```python
from build123d import *

# Parameters (mm, degrees)
SKETCH3_R           = 3
CUT_EXTRUDE1_DEPTH  = 1.5
SKETCH4_R           = 1.5
CUT_EXTRUDE2_DEPTH  = 2.5
SKETCH5_R           = 5
SKETCH5_R_2         = 4
EXTRUDE_THIN1_DEPTH = 2


with BuildPart() as part:
    # Sketch1 → Revolve1 (revolve)
    with BuildSketch(Plane(origin=(0, 0, 0), x_dir=(1, 0, 0), z_dir=(0, 1, 0))):
        Polygon((0, -1), (4.5, -1), (4.5, 0), (7.5, 0), (7.5, -1), (14, -1), (14, 1), (15, 1), (15, 2), (0, 2), align=None)
    revolve(axis=Axis((0, 0, -2), (0, 0, 1)))

    # Sketch3 → Cut-Extrude1 (cut)
    with BuildSketch(Plane.XY.offset(1)):
        Circle(SKETCH3_R)
    extrude(amount=-CUT_EXTRUDE1_DEPTH, mode=Mode.SUBTRACT)

    # Sketch4 → Cut-Extrude2 (cut, through all)
    with BuildSketch(Plane.XY.offset(-0.5)):
        Circle(SKETCH4_R)
    extrude(amount=-CUT_EXTRUDE2_DEPTH, mode=Mode.SUBTRACT)

    # Sketch5 → Extrude-Thin1 (add)
    with BuildSketch(Plane(origin=(0, 0, -2), x_dir=(-1, 0, 0), z_dir=(0, 0, -1))):
        Circle(SKETCH5_R)
        Circle(SKETCH5_R_2, mode=Mode.SUBTRACT)
    extrude(amount=EXTRUDE_THIN1_DEPTH)


solid = part.part
```
Check sheet for the modelled part. Datum: model origin and axes. Units: mm. A direction names the side the tool comes from. Round coordinates to 2 decimals unless told otherwise and drop trailing zeros. Loops run counter-clockwise (first coordinate to the right, second up) from the corner with the lowest first, then second, coordinate; pieces in that order, holes last. Notation, with made-up numbers: (11.5, 1) - (34.5, 1) arc R20 ccw to (34.5, 23) - close; hole circle Ø1 at (41, 11.25). An arc over 180 degrees is marked (long way). Answer as a JSON object with one key per item and string values. Group by question number.
Q1. Sectioned sample at D-D, the plane x = 12. Enter the section's corners in (y, z).
Q2. Mould release check, pull along X, two halves, no side actions. Record for faces 1 (the face through (1.08, -4.88, -2.99)), 2 (the face through (-1.5, 0.07, -1.24)), 3 (the face through (0, -5, 0)), 4 (the face through (-4, 4, -2)): released by +X, released by -X, zero draft, split by the parting line, or undercut.
Q3. Set-up check for faces 5 (the face through (0.867, -3.905, -2.986)), 6 (the face through (-0.59, 4.46, 0.49)), 7 (the face through (-1, -3, 1)): record each of +Z, -Z, +X, -X, +Y, -Y from which the full face is reachable in a straight line by a thin tool's end or side.
Q4. Scan lines: line 1 along Y through (x, z) = (0, 0.3); line 2 along Y through (x, z) = (0, -1.05); line 3 along Y through (x, z) = (0, -3.1). Record each from-to range of solid material in increasing order. Write a range as [from, to].
Q5. Sectioned sample at C-C, the plane z = -3.05. Enter the section's corners in (x, y).
Q6. Gauge pin test, flat ends, axial feed: P1, Ø5, axis at x = 0, y = 0, coming from the +Z side; P2, Ø3, axis at y = 9.5, z = -1, coming from the -X side; P3, Ø2.5, axis at x = -1, y = -0.5, coming from the -Z side; P4, Ø1.5, axis at x = -7, z = -3, coming from the +Y side. Record the tip position at first contact, or that the pin passes through.
Solution:
{
 "1": {"outline": "(-9, -2) - (9, -2) - (9, -1) - (7.21, -1) - (7.21, 1) - (-7.21, 1) - (-7.21, -1) - (-9, -1) - close"},
 "2": {"face 1": "split by the parting line", "face 2": "undercut", "face 3": "undercut", "face 4": "zero draft"},
 "3": {"face 5": "-Z", "face 6": "+Z", "face 7": "+Z, +X, -X, +Y, -Y"},
 "4": {"line 1": "y = [-14, -7.5], [-4.5, -3], [3, 4.5], [7.5, 14]", "line 2": "y = [-15, -1.5], [1.5, 15]", "line 3": "y = [-5, -4], [4, 5]"},
 "5": {"outline": "circle Ø10 at (0, 0); hole circle Ø8 at (0, 0)"},
 "6": {"P1": "stops at z = -0.5", "P2": "stops at x = -12.69", "P3": "stops at z = -2", "P4": "passes through"}
}
